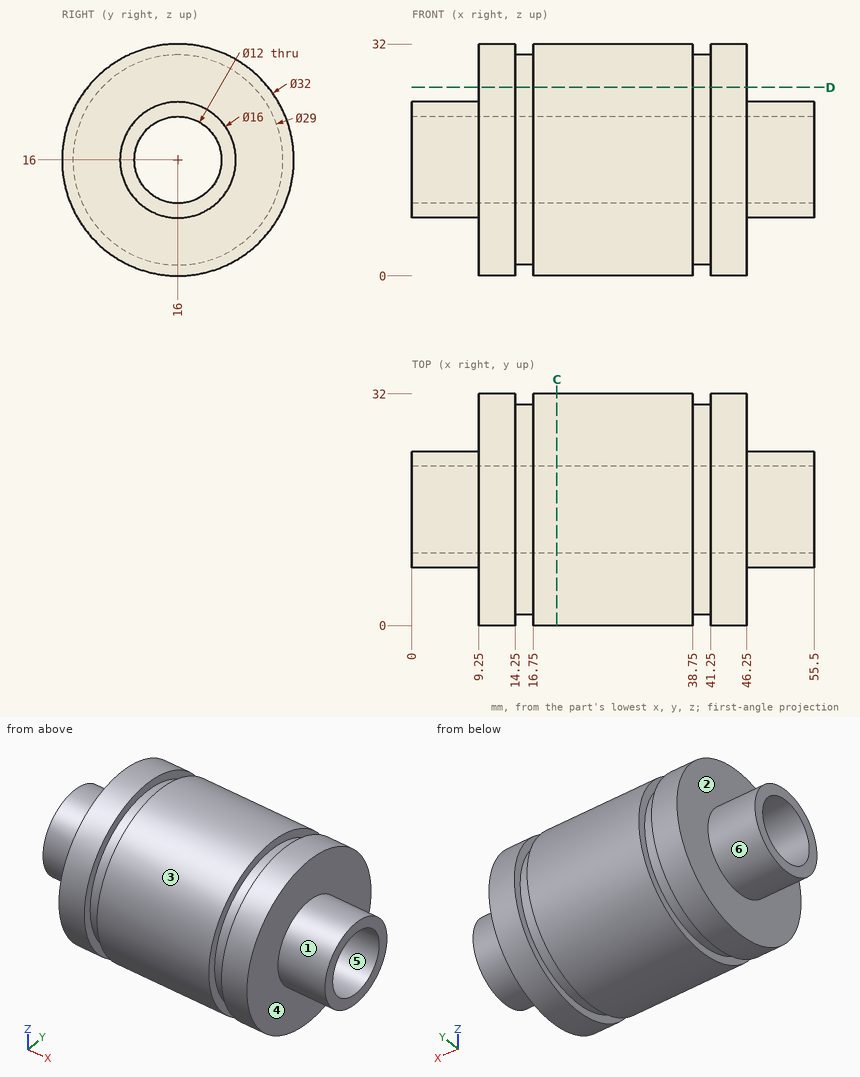
Answer from the drawing. Dimensions are ordinates in mm from the lowest x, y and z of the part. A direction names the side the tool comes from. Round coordinates to 2 decimals unless told otherwise and drop trailing zeros. Order: outer loops, then holes, each group sorted by start corner. A loop starts at its lowest first (then second) coordinate and runs counter-clockwise, first axis right, second up. Notation, with made-up numbers: (-16, -16) -> (6, -16) arc R35 ccw to (6, 20) -> close; hole circle Ø2 at (3, 56.25). An arc over 180 degrees is marked (long way). Answer as CSV lines item,"result".
Q1. A cutting plane is placed at D-D on z = 26. Determine the outline of the cut face in (x, y).
Computed values:
outline,"(9.25, 3.51) -> (14.25, 3.51) -> (14.25, 5.5) -> (16.75, 5.5) -> (16.75, 3.51) -> (38.75, 3.51) -> (38.75, 5.5) -> (41.25, 5.5) -> (41.25, 3.51) -> (46.25, 3.51) -> (46.25, 28.49) -> (41.25, 28.49) -> (41.25, 26.5) -> (38.75, 26.5) -> (38.75, 28.49) -> (16.75, 28.49) -> (16.75, 26.5) -> (14.25, 26.5) -> (14.25, 28.49) -> (9.25, 28.49) -> close"
Q2. Which of the six approach directions +Z, -Z, +X, -X, +Y, -Y give full straight-line access (tool end or side, diameter ignored) to the marked faces 1, 2 and 3?
Computed values:
face 1,"+X"
face 2,"-X"
face 3,"+X, -X"
Q3. Consider line 1 (X direction, y = 24, z = 28.5); line 2 (Y direction, x = 25.5, z = 16); line 3 (X direction, y = 20.5, z = 26). Determine where each line is inside the solid, lowest interval first. Write a range as from..to.
Computed values:
line 1,"x = 9.25..14.25, 16.75..38.75, 41.25..46.25"
line 2,"y = 0..10, 22..32"
line 3,"x = 9.25..46.25"
Q4. Given pin 1 (4 mm diameter, centred on x = 34.5, z = 20.5, fed in from -Y); pin 2 (2 mm diameter, centred on x = 43, z = 5.5, fed in from +Y); pin 3 (8 mm diameter, centred on x = 33.5, y = 6, fed in from -Z); pin 4 (9.5 mm diameter, centred on y = 12, z = 18.5, fed in from -X), each flat-ended and moving along its own axis, determine where each tip first touches the part or whether it passes through.
Computed values:
pin 1,"stops at y = 0.2"
pin 2,"stops at y = 28.87"
pin 3,"stops at z = 1.17"
pin 4,"stops at x = 0"
Q5. A cutting plane is placed at C-C on x = 20. Determine the outline of the cut face in (y, z), plus the area to 3 significant figures.
Computed values:
outline,"circle Ø32 at (16, 16); hole circle Ø12 at (16, 16)"
area,"691 mm^2"
Q6. For a pull along Y with two mould halves and no side action, classify the marked faces 4, 5 and 6 as +Y half, -Y half, draft (parallel to the pull), parting line (faces both ways), or undercut.
Computed values:
face 4,"draft"
face 5,"undercut"
face 6,"parting line"
